from build123d import *

# Parameters (mm, degrees)
PAD009_DEPTH      = 10
PAD009_DEPTH_BACK = 10
SKETCH_W          = 4
SKETCH_H          = 7.426
PAD008_DEPTH      = 1
SKETCH007_R       = 3.35
PAD007_DEPTH      = 1.5
SKETCH006_W       = 5.4
SKETCH006_H       = 5.4
PAD006_DEPTH      = 5
SKETCH001_W       = 9.6
SKETCH001_H       = 9.22
PAD_DEPTH         = 1.3
PAD_DEPTH_BACK    = 0.25


with BuildPart() as bottom_cut_avoid_thin_bridge:
    # Sketch008 → Pad009 (new body, two sides)
    with BuildSketch(Plane.XY) as pad009_sk:
        with BuildLine():
            Line((-1.982914, -2.691867), (1.982914, -2.691867))
            add(Edge.make_bspline(
                [(1.982914, -2.691867), (1.306801, -3.14996), (0.04804, -3.514381), (-1.402881, -3.141278), (-1.982914, -2.691867)],
                knots=[0, 0, 0, 0, 0.5, 1, 1, 1, 1], degree=3))
        make_face()
    extrude(amount=PAD009_DEPTH)
    extrude(pad009_sk.sketch, amount=-PAD009_DEPTH_BACK)


with BuildPart() as sensor_entrance_channel_cut:
    # Sketch → Pad008 (new body)
    with BuildSketch(Plane.XY):
        with Locations((0, -1.787)):
            Rectangle(SKETCH_W, SKETCH_H)
    extrude(amount=-PAD008_DEPTH)


with BuildPart() as o_ring_cutout:
    # Sketch007 → Pad007 (new body)
    with BuildSketch(Plane.XY):
        Circle(SKETCH007_R)
    extrude(amount=PAD007_DEPTH)


with BuildPart() as o_ring_cutout_1:
    # Body007 placement: moved
    add(o_ring_cutout.part.moved(Location((0, 0, 0.65))))


with BuildPart() as glass_cutout:
    # Sketch006 → Pad006 (new body)
    with BuildSketch(Plane.XY):
        Rectangle(SKETCH006_W, SKETCH006_H)
    extrude(amount=PAD006_DEPTH)


with BuildPart() as cut003:
    # Sketch001 → Pad (new body, two sides)
    with BuildSketch(Plane.XY) as pad_sk:
        with Locations((0, -0.61)):
            Rectangle(SKETCH001_W, SKETCH001_H)
    extrude(amount=PAD_DEPTH)
    extrude(pad_sk.sketch, amount=-PAD_DEPTH_BACK)


with BuildPart() as cut003_1:
    # Body001 placement: moved
    add(cut003.part.moved(Location((0, 0.5, 0))))

    # Cut: cut Glass _cutout
    add(glass_cutout.part, mode=Mode.SUBTRACT)

    # Cut001: cut O-ring_Cutout
    add(o_ring_cutout_1.part, mode=Mode.SUBTRACT)

    # Cut002: cut sensor entrance channel cut
    add(sensor_entrance_channel_cut.part, mode=Mode.SUBTRACT)

    # Cut003: cut Bottom_Cut_avoid_thin_bridge
    add(bottom_cut_avoid_thin_bridge.part, mode=Mode.SUBTRACT)


solid = cut003_1.part
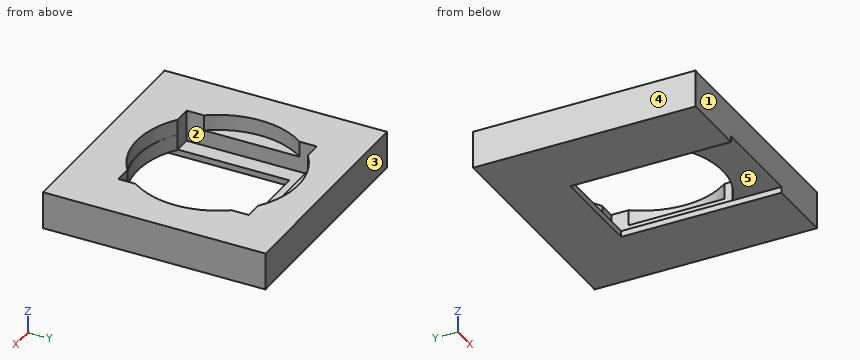
Could you check a few things on this model? Use its own coordinates, in mm. Face numbers are marked on the shaded views. A direction names the side the tool comes from. Coordinates: 2 decimals unless noted, no trailing zeros. Loops run counter-clockwise (first coordinate to the right, second up) from the corner with the lowest first, then second, coordinate; pieces in that order, holes last. Notation, with made-up numbers: (45.25, 19) -> (92.25, 19) arc R26 cw to (92.25, 44) -> close; hole circle Ø2 at (-23.5, 39). An arc over 180 degrees is marked (long way). Answer in a Markdown table with one row per item.
(1) Imagine slicing it at A-A (y = -2.25). List the corners of the cut face in (x, z) for me, plus the area to 3 significant figures.
Results found:
| item | result |
|---|---|
| outline | (-4.8, -0.25) -> (-2, -0.25) -> (-2, 0) -> (-2.7, 0) -> (-2.7, 1.3) -> (-4.8, 1.3) -> close; (2, -0.25) -> (4.8, -0.25) -> (4.8, 1.3) -> (2.7, 1.3) -> (2.7, 0) -> (2, 0) -> close |
| area | 6.86 mm^2 |
(2) Thinking about a two-plate mould opening in X: for the marked faces 3, 4 and 5, which applies, released by +X, released by -X, zero draft, split by the parting line, or undercut?
Results found:
| item | result |
|---|---|
| face 3 | zero draft |
| face 4 | released by -X |
| face 5 | undercut |
(3) If I drill on probe 1 along X at (y, z) = (0.75, 0.5); probe 2 along Y at (x, z) = (0, 0.45); probe 3 along Z at (x, y) = (-2.5, -0.25), over which ranges is the centre line in solid material (lowest first)?
Results found:
| item | result |
|---|---|
| probe 1 | x = -4.8 to -2.7, 2.7 to 4.8 |
| probe 2 | y = -4.72 to -3.33, 2.7 to 4.5 |
| probe 3 | z = -0.25 to 0 |
(4) Imagine slicing it at C-C (x = -2.5). List the corners of the cut face in (y, z) for me.
Results found:
| item | result |
|---|---|
| outline | (-4.72, -0.25) -> (4.5, -0.25) -> (4.5, 1.3) -> (2.7, 1.3) -> (2.7, 0) -> (-2.7, 0) -> (-2.7, 1.3) -> (-4.72, 1.3) -> close |
(5) Imagine slicing it at D-D (y = -3.5). List the corners of the cut face in (x, z) for me.
Results found:
| item | result |
|---|---|
| outline | (-4.8, -0.25) -> (-2, -0.25) -> (-2, 0) -> (2, 0) -> (2, -0.25) -> (4.8, -0.25) -> (4.8, 1.3) -> (-4.8, 1.3) -> close |
(6) Will these pins go through, and if not, where does the flat tip stop? pin 1 Ø4.5 at (x, y) = (0, 1) entering from +Z; pin 2 Ø1 at (x, y) = (-1, -3.5) entering from -Z.
Results found:
| item | result |
|---|---|
| pin 1 | stops at z = 0.65 |
| pin 2 | stops at z = 0 |
(7) For the marked faces 1 and 2, which set-ups out of +Z, -Z, +X, -X, +Y, -Y let a thin tool reach every point of the face, with its end or its side?
Results found:
| item | result |
|---|---|
| face 1 | +Z, -Z, +X, -X, -Y |
| face 2 | +Z |
(8) Imagine slicing it at B-B (z = 1.15). List the corners of the cut face in (x, y) for me, plus the area to 3 significant figures.
Results found:
| item | result |
|---|---|
| outline | (-4.8, -4.72) -> (4.8, -4.72) -> (4.8, 4.5) -> (-4.8, 4.5) -> close; hole (-2.7, -2.7) -> (-1.98, -2.7) arc R3.35 ccw to (1.98, -2.7) -> (2.7, -2.7) -> (2.7, -1.98) arc R3.35 ccw to (2.7, 1.98) -> (2.7, 2.7) -> (1.98, 2.7) arc R3.35 ccw to (-1.98, 2.7) -> (-2.7, 2.7) -> (-2.7, 1.98) arc R3.35 ccw to (-2.7, -1.98) -> close |
| area | 52.3 mm^2 |
